Autodesk Fusion 360 part; units mm, degrees
sketch "Sketch1" plane through (0, 0, 0) normal (0, 0, 1) x (1, 0, 0)
  line L0 (-0.85, -0.0168) -> (-0.85, 9) construction
  line L1 (6.85, -0.0176) -> (6.85, 9) construction
  line L2 (1.7299, 0) -> (1.7299, 2.58) construction
  line L3 (4.2701, 0) -> (4.2701, 2.58) construction
  line L4 (4.2701, 0) -> (4.2701, -2.58) construction
  line L5 (1.7299, 0) -> (1.7299, -2.58) construction
  line L6 (4.2701, 2.58) -> (1.7299, 2.58)
  line L7 (3, 2.2457) -> (3, -2.58) construction
  arc A0 (1.7299, 2.58) -> (1.7299, -2.58) centre (1.7299, 0) ccw
  arc A1 (4.2701, -2.58) -> (4.2701, 2.58) centre (4.2701, 0) ccw
  line L8 (1.7299, -1.545) -> (1.7299, -2.58)
  line L9 (4.2701, -1.545) -> (4.2701, -2.58)
  arc A2 (4.2701, -1.545) -> (1.7299, -1.545) centre (3, 0) ccw
  dimension "d3" = 7.7
  dimension "d4" = 4
extrude "Extrude1" add sketch "Sketch1" along normal blind 2.7
Could you check a few things on this model? Use its own coordinates, in mm. A direction names the side the tool comes from. Coordinates: 2 decimals unless noted, no trailing zeros. Order: outer loops, then holes, each group sorted by start corner. A loop starts at its lowest first (then second) coordinate and runs counter-clockwise, first axis right, second up.
Q1. Please list where these lines run through material, in increasing order: L1, parallel to X at y = 0, z = 0.8; L2, parallel to X at y = 1.5, z = 2.15; L3, parallel to Y at x = 1.25, z = 2.
Q2. Suppose I cut it at A-A on y = 0. Please give me the cut outline in (x, z).
Q3. Suppose I cut it at D-D on x = 3. Please give me the cut outline in (y, z), and give its area (3 significant figures).
Q4. Suppose I cut it at C-C on z = 1.7. Please give me the cut outline in (x, y) (3 decimals).
Q5. Thinking about a two-plate mould opening in X: for faces 3 (the flat face through (3, 2.58, 1)), 4 (the cylindrical face through (-0.85, -0.06, 1.33)), 5 (the flat face through (1.73, -2, 1)), which applies, released by +X, released by -X, zero draft, split by the parting line, or undercut?
Q6. Which directions (+Z, -Z, +X, -X, +Y, -Y) give clear straight access to the entire face, cutting with the end or side of a thin tool? Please do faces 1 (the flat face through (4.27, -2, 1)), 2 (the cylindrical face through (3, 2, 1)).
Q7. Will these pins go through, and if not, where does the flat tip stop? pin 1 (1.1 mm diameter, centred on y = -2, z = 1, fed in from +X); pin 2 (1 mm diameter, centred on y = -1.5, z = 2, fed in from +X); pin 3 (0.5 mm diameter, centred on y = -2.5, z = 1.5, fed in from -X).
Q8. Suppose I cut it at B-B on x = 4.75. Please give me the cut outline in (y, z).
Answer:
1. L1: x = -0.85 to 1, 5 to 6.85
1. L2: x = -0.37 to 1.68, 4.32 to 6.37
1. L3: y = -2.53 to -0.97, 0.97 to 2.53
2. outline: (-0.85, 0) - (1, 0) - (1, 2.7) - (-0.85, 2.7) - close; (5, 0) - (6.85, 0) - (6.85, 2.7) - (5, 2.7) - close
3. outline: (2, 0) - (2.58, 0) - (2.58, 2.7) - (2, 2.7) - close
3. area: 1.57 mm2
4. outline: (1.73, -2.58) - (1.73, -1.545) arc R2 cw (long way) to (4.27, -1.545) - (4.27, -2.58) arc R2.58 ccw to (4.27, 2.58) - (1.73, 2.58) arc R2.58 ccw to start
5. face 3: zero draft
5. face 4: released by -X
5. face 5: undercut
6. face 1: +Z, -Z, -Y
6. face 2: +Z, -Z
7. pin 1: stops at x = 6.4
7. pin 2: stops at x = 6.65
7. pin 3: stops at x = 0.47
8. outline: (-2.53, 0) - (-0.97, 0) - (-0.97, 2.7) - (-2.53, 2.7) - close; (0.97, 0) - (2.53, 0) - (2.53, 2.7) - (0.97, 2.7) - close
